Source: three-view drawing plus pictorial views. Frame: mm from the lowest corner of the part. Give positions to 0.01 mm unless a question says otherwise; leave off trailing zeros. Order: outer loops, then holes, each group sorted by start corner. A loop starts at its lowest first (then second) coordinate and runs counter-clockwise, first axis right, second up. Notation, with made-up numbers: (78.25, 27) - (93.25, 27) arc R25 cw to (93.25, 62) - close; hole circle Ø5 at (83.5, 41). An arc over 180 degrees is marked (long way). Answer in a Markdown table with one row per item. Add a question column.
1. Section query D-D on z = 20. Return loops of the section in (x, y).
2. Ray query, line 1 (X direction, y = 3.5, z = 115.5); line 2 (X direction, y = 8.25, z = 20); line 3 (X direction, y = 1, z = 58). Return the intervals inside material, ascending. Write a range as [from, to].
3. Contact query for a flat-ended pin moving along its axis: pin 1 (3.5 mm diameter, centred on x = 107.75, z = 83.5, fed in from -Y). Output: stop coordinate, or through.
4. Section query B-B on y = 5.5. Count the separate pieces of the cut face and the enclosed holes in it, and give its area (3 significant figures).
5. Section query C-C on z = 163. Return loops of the section in (x, y), and give its area (3 significant figures).
6. Section query A-A on x = 125. Return loops of the section in (y, z), and give its area (3 significant figures).
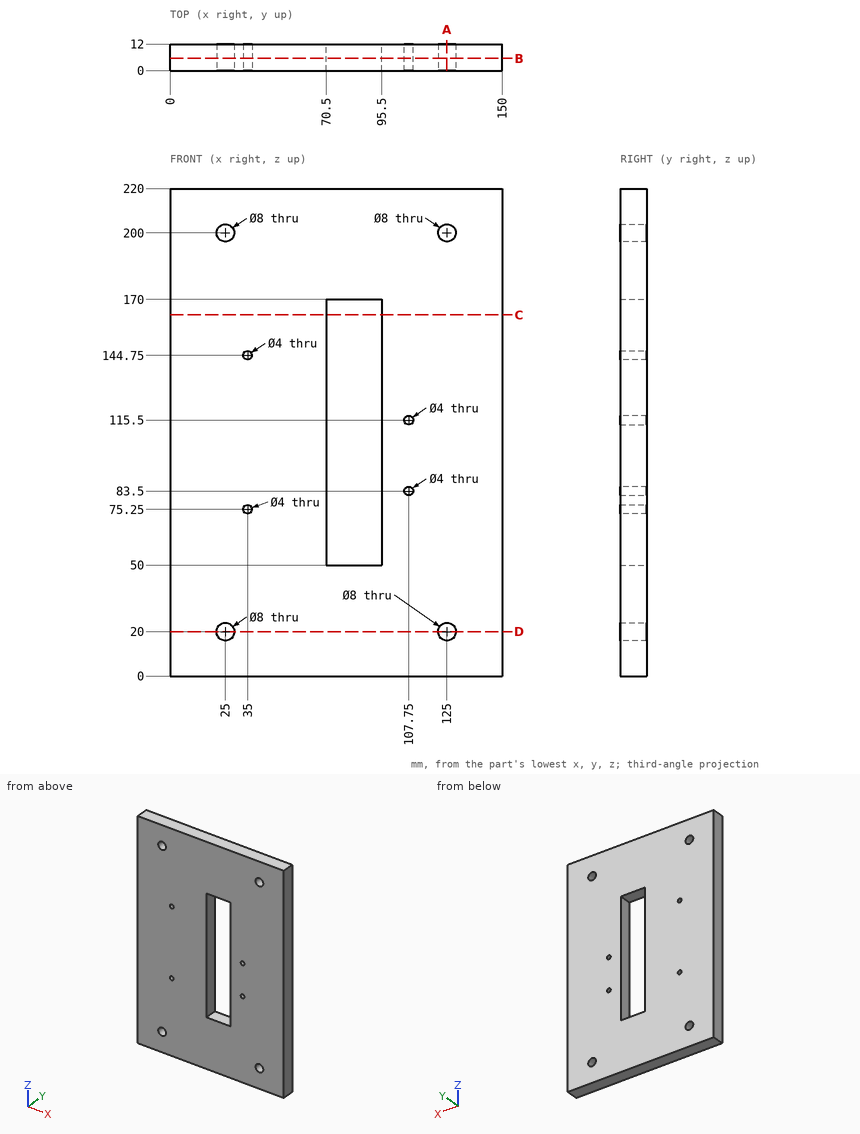
Answer:
| question | item | result |
|---|---|---|
| 1 | outline | (0, 0) - (21, 0) - (21, 12) - (0, 12) - close; (29, 0) - (121, 0) - (121, 12) - (29, 12) - close; (129, 0) - (150, 0) - (150, 12) - (129, 12) - close |
| 2 | line 1 | x = [0, 70.5], [95.5, 105.75], [109.75, 150] |
| 2 | line 2 | x = [0, 21], [29, 121], [129, 150] |
| 2 | line 3 | x = [0, 70.5], [95.5, 150] |
| 3 | pin 1 | passes through |
| 4 | separate pieces | 1 |
| 4 | enclosed holes | 9 |
| 4 | area | 29,700 mm² |
| 5 | outline | (0, 0) - (70.5, 0) - (70.5, 12) - (0, 12) - close; (95.5, 0) - (150, 0) - (150, 12) - (95.5, 12) - close |
| 5 | area | 1,500 mm² |
| 6 | outline | (0, 0) - (12, 0) - (12, 16) - (0, 16) - close; (0, 24) - (12, 24) - (12, 196) - (0, 196) - close; (0, 204) - (12, 204) - (12, 220) - (0, 220) - close |
| 6 | area | 2,450 mm² |
